```python
from build123d import *

# Parameters (mm, degrees)
F0_R     = 12.065
F1_DEPTH = 50.8
F2_R     = 1.8415
F3_DEPTH = 12.7
F4_SIZE  = 10.16


with BuildPart() as f1:
    # F0 (on Right) → F1 (new body)
    with BuildSketch(Plane.YZ):
        with Locations((-32.940101, 30.467385)):
            Circle(F0_R)
    extrude(amount=F1_DEPTH)

    # F2 (on face) → F3 (join)
    with BuildSketch(Plane.YZ.offset(50.8)):
        with Locations((-32.940101, 30.467385)):
            Circle(F2_R)
    extrude(amount=F3_DEPTH)

    # F4
    f4_edges = [f1.edges().sort_by_distance(p)[0] for p in [
        (50.8, -45.005101, 30.467385),
    ]]
    chamfer(f4_edges, length=F4_SIZE)


solid = f1.part
```
The listing builds one solid part. Answer for the finished solid, in the listing's coordinates (mm). A direction names the side the tool comes from. Coordinates: 2 decimals unless noted, no trailing zeros. Loops run counter-clockwise (first coordinate to the right, second up) from the corner with the lowest first, then second, coordinate; pieces in that order, holes last. Notation, with made-up numbers: (-6.75, 1.25) -> (38.25, 1.25) arc R19 cw to (38.25, 12.25) -> close; hole circle Ø8 at (-11, 10.25). An arc over 180 degrees is marked (long way). Return JSON: item names as keys, results as strings. Group by question number.
(1) A cutting plane is placed at A-A on x = 21. Write down the section's boundary in (y, z) (3 decimals).
(2) Given pin 1 Ø6 at (x, y) = (39, -26.5) entering from -Z; pin 2 Ø1 at (y, z) = (-37.5, 36) entering from +X; pin 3 Ø10 at (y, z) = (-25.5, 36.5) entering from +X; pin 4 Ø1.5 at (x, z) = (46, 39) entering from +Y, each flat-ended and moving along its own axis, determine where each tip first touches the part or whether it passes through.
(3) Find the intervals of material crossed by probe 1 along Z at (x, y) = (4.5, -33); probe 2 along X at (y, z) = (-29, 33.5); probe 3 along Z at (x, y) = (34, -25.25), in increasing order. Write a range as from..to.
(4) Which of the six approach directions +Z, -Z, +X, -X, +Y, -Y give full straight-line access (tool end or side, diameter ignored) to faces 1 (the cylindrical face through (20.04, -26.45, 40.64)), 2 (the cylindrical face through (57.06, -34.78, 30.55))?
(5) A cutting plane is placed at B-B on x = 48. Write down the section's boundary in (y, z) (3 decimals).
The answers:
{
 "1": {"outline": "circle Ø24.13 at (-32.94, 30.467)"},
 "2": {"pin 1": "stops at z = 18.9", "pin 2": "stops at x = 46.04", "pin 3": "stops at x = 48.13", "pin 4": "passes through"},
 "3": {"probe 1": "z = 18.4..42.53", "probe 2": "x = 0..47.73", "probe 3": "z = 21.17..39.76"},
 "4": {"face 1": "+X, -X", "face 2": "+X"},
 "5": {"outline": "circle Ø9.41 at (-32.94, 30.467)"}
}
